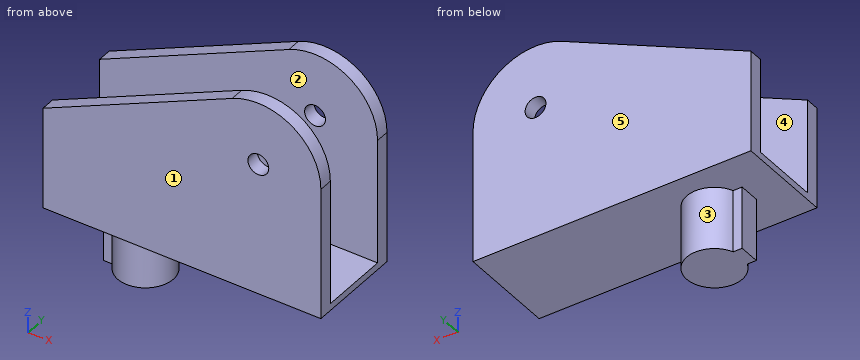
```python
from build123d import *

# Parameters (mm, degrees)
SKETCH_1_R          = 7.5
EXTRUDE_1_DEPTH     = 10
SKETCH_3_W          = 5
SKETCH_3_H          = 35
EXTRUDE_2_DEPTH     = 200
EXTRUDE_START       = -60
SKETCH_1_2_R        = 7.5
EXTRUDE_3_DEPTH     = 60
SKETCH_7_W          = 135
SKETCH_7_H          = 50
CUT_EXTRUDE_1_DEPTH = 230.401394939
EXTRUDE_4_DEPTH     = 45


with BuildPart() as part:
    # 草图1 → 凸台-拉伸1 (new body)
    with BuildSketch(Plane(origin=(0, 0, 0), x_dir=(1, 0, 0), z_dir=(0, 1, 0))):
        with BuildLine():
            Line((45, 0), (45, 90))
            Line((45, 90), (-155, 90))
            Line((-155, 90), (-155, 21.804554274))
            Line((-155, 21.804554274), (-18.814985094, -40.877822054))
            ThreePointArc((-18.814985094, -40.877822054), (24.272676725, -37.892442051), (45, 0))
        make_face()
        with Locations(Location((0, 0, 0), (0, 0, 270))):
            Circle(SKETCH_1_R, mode=Mode.SUBTRACT)
    extrude(amount=EXTRUDE_1_DEPTH)

    # 草图3 → 凸台-拉伸2 (add)
    with BuildSketch(Plane(origin=(45, 0, 0), x_dir=(0, 0, -1), z_dir=(1, 0, 0))):
        with Locations((92.5, -7.5)):
            Rectangle(SKETCH_3_W, SKETCH_3_H)
    extrude_2 = extrude(amount=-EXTRUDE_2_DEPTH)

    # 镜向5: 凸台-拉伸2 across plane
    add(extrude_2.mirror(Plane(origin=(0, -25, 0), x_dir=(0, 0, 1), z_dir=(0, -1, 0))))

    # 草图1<2> → 凸台-拉伸3 (add)
    with BuildSketch(Plane(origin=(0, 0, 0), x_dir=(1, 0, 0), z_dir=(0, 1, 0)).offset(EXTRUDE_START)):
        with BuildLine():
            Line((45, 0), (45, 90))
            Line((45, 90), (-155, 90))
            Line((-155, 90), (-155, 21.804554274))
            Line((-155, 21.804554274), (-18.814985094, -40.877822054))
            ThreePointArc((-18.814985094, -40.877822054), (24.272676725, -37.892442051), (45, 0))
        make_face()
        with Locations(Location((0, 0, 0), (0, 0, 90))):
            Circle(SKETCH_1_2_R, mode=Mode.SUBTRACT)
    extrude(amount=EXTRUDE_3_DEPTH)

    # 草图7 → 切除-拉伸1 (cut, through all)
    with BuildSketch(Plane(origin=(45, 0, 0), x_dir=(0, 0, -1), z_dir=(1, 0, 0))):
        with Locations((22.5, -25)):
            Rectangle(SKETCH_7_W, SKETCH_7_H)
    extrude(amount=-CUT_EXTRUDE_1_DEPTH, mode=Mode.SUBTRACT)

    # 草图8 → 凸台-拉伸4 (add)
    with BuildSketch(Plane(origin=(0, 0, -95), x_dir=(-1, 0, 0), z_dir=(0, 0, -1))):
        with BuildLine():
            Line((123.540496218, -17.5), (130, -17.5))
            Line((130, -17.5), (130, -32.5))
            Line((130, -32.5), (123.540496218, -32.5))
            ThreePointArc((123.540496218, -32.5), (85, -25), (123.540496218, -17.5))
        make_face()
    extrude(amount=EXTRUDE_4_DEPTH)


solid = part.part
```
The listing builds one solid part. Answer for the finished solid, in the listing's coordinates (mm). Face numbers are marked on the shaded views. A direction names the side the tool comes from. Give positions to 0.01 mm unless a question says otherwise; leave off trailing zeros. Write each loop counter-clockwise with the first axis right and the second up, starting at its lowest first coordinate (ties: lowest second). Pieces come first, ordered by that corner, then holes. Notation, with made-up numbers: (88.5, -37) -> (125.5, -37) arc R16 cw to (125.5, -25) -> close; hole circle Ø3 at (79, 17.25). An arc over 180 degrees is marked (long way). Write item = value, one per line. Start each with the question number.
1) The part is cut by section C-C, the plane y = -20. Determine the outline of the cut face in (x, z).
2) Which of the six approach directions +Z, -Z, +X, -X, +Y, -Y give full straight-line access (tool end or side, diameter ignored) to the marked faces 4 and 5?
3) Each of these flat-tipped pins is pushed along its axis until it touches: pin 1 (1.9 mm diameter, centred on x = -126, z = -116.5, fed in from +Y); pin 2 (5 mm diameter, centred on x = -53.5, y = -20.5, fed in from +Z); pin 3 (16.5 mm diameter, centred on y = -23, z = -112, fed in from -X). Where does it stop, or does it pass through?
4) Straight lines are drawn through the part: line 1 along Y through (x, z) = (-118, -54); line 2 along X through (y, z) = (4.5, 0); line 3 along Z through (x, y) = (-111.5, -48). For each, find the intervals that lie inside material, in ascending order.
5) Determine the mould class of the marked faces 1, 2 and 3 for opening direction Y: +Y half, -Y half, draft (parallel to the pull), parting line (faces both ways), or undercut.
6) The part is cut by section A-A, the plane z = -69. Determine the outline of the cut face in (x, y).
7) The part is cut by section B-B, the plane x = 0. Determine the outline of the cut face in (y, z).
8) The part is cut by section D-D, the plane z = 24.5. Determine the outline of the cut face in (x, y), and give its area (3 significant figures).
Solutions:
q1.outline = (-155, -95) -> (-130, -95) -> (-130, -140) -> (-85.64, -140) -> (-85.64, -95) -> (45, -95) -> (45, -90) -> (-155, -90) -> close
q2.face_4 = +Z, +X, -X
q2.face_5 = +Z, -Z, +X, -X, +Y
q3.pin_1 = -17.5
q3.pin_2 = -90
q3.pin_3 = -130
q4.line_1 = -60 to -50, 0 to 10
q4.line_2 = -107.63 to -7.5, 7.5 to 45
q4.line_3 = -95 to -90
q5.face_1 = -Y half
q5.face_2 = undercut
q5.face_3 = parting line
q6.outline = (-155, -60) -> (45, -60) -> (45, -50) -> (-155, -50) -> close; (-155, 0) -> (45, 0) -> (45, 10) -> (-155, 10) -> close
q7.outline = (-60, -95) -> (10, -95) -> (10, -7.5) -> (0, -7.5) -> (0, -90) -> (-50, -90) -> (-50, -7.5) -> (-60, -7.5) -> close; (-60, 7.5) -> (-50, 7.5) -> (-50, 45) -> (-60, 45) -> close; (0, 7.5) -> (10, 7.5) -> (10, 45) -> (0, 45) -> close
q8.outline = (-54.4, -60) -> (37.75, -60) -> (37.75, -50) -> (-54.4, -50) -> close; (-54.4, 0) -> (37.75, 0) -> (37.75, 10) -> (-54.4, 10) -> close
q8.area = 1,840 mm²
